Geometry check sheet. Reference: the model listing, model coordinates, mm. A direction names the side the tool comes from. Give positions to 0.01 mm unless a question says otherwise; leave off trailing zeros. Loops run counter-clockwise (first coordinate to the right, second up) from the corner with the lowest first, then second, coordinate; pieces in that order, holes last. Notation, with made-up numbers: (-26, 38.25) -> (22, 38.25) arc R11 ccw to (22, 52.25) -> close; hole circle Ø3 at (81, -34). An arc over 180 degrees is marked (long way). Write each question's results on one line, items separated by ' | '. Start each with the question number.
1) Sectioned sample at B-B on x = -2.5. Record the cut outline in (y, z).
2) Set-up check for faces 1 (the face through (3, 8, 6)), 2 (the face through (-3, 40.514, 6)), 3 (the face through (-3, 40.514, -6)), 4 (the face through (3, 40.514, 6)): record each of +Z, -Z, +X, -X, +Y, -Y from which the full face is reachable in a straight line by a thin tool's end or side.
3) Depth check by flat-ended pin: pin 1 (3 mm diameter, centred on y = 41.5, z = 1, fed in from +X); pin 2 (1 mm diameter, centred on x = -5.5, y = 10.5, fed in from +Z); pin 3 (3 mm diameter, centred on y = 24.5, z = 4.5, fed in from -X). Enter the tip coordinate at first touch or a pass-through.
4) Scan lines: line 1 (X direction, y = 38, z = -4.5); line 2 (X direction, y = 43, z = -3.5); line 3 (Z direction, x = 4.5, y = 7). Record each from-to range of solid material in increasing order. Write a range as from..to.
5) Sectioned sample at A-A on z = -2.5. Record the cut outline in (x, y), then the cut area to 3 significant figures.
6) Sectioned sample at C-C on y = 22. Record the cut outline in (x, z).
Autodesk Inventor part; units mm, degrees
ref_plane "Work Plane2" through (0, 24.257, 0) normal (0, 1, 0) x (1, 0, 0)
ref_plane "YZ Plane" through (0, 0, 0) normal (1, 0, 0) x (0, 1, 0)
ref_plane "XZ Plane" through (0, 0, 0) normal (0, 1, 0) x (-1, 0, 0)
sketch "Sketch1" plane through (0, 0, 0) normal (0, 1, 0) x (-1, 0, 0)
  line L0 (7.3323, 0) -> (3.6662, -6.35)
  line L1 (3.6662, -6.35) -> (-3.6662, -6.35)
  line L2 (-3.6662, -6.35) -> (-7.3323, 0)
  line L3 (-7.3323, 0) -> (-3.6662, 6.35)
  line L4 (-3.6662, 6.35) -> (3.6662, 6.35)
  line L5 (3.6662, 6.35) -> (7.3323, 0)
  line L6 (7.3323, 0) -> (0, 0)
  line L7 (0, 0) -> (0, -3.7196)
  dimension "d0" = 90
  dimension "d1" = 12.7
extrude "Extrusion1" add sketch "Sketch1" along normal blind 48.514
ref_plane "Work Plane2" through (0, 24.257, 0) normal (0, 1, 0) x (1, 0, 0)
sketch "Sketch3" plane through (0, 48.514, 0) normal (0, 1, 0) x (1, 0, 0)
  circle A0 centre (0, 0) radius 6.35
  line L0 (-3.6662, 6.35) -> (-7.3323, 0)
  line L1 (-3.6662, 6.35) -> (-7.3323, 0)
  line L2 (-7.3323, 0) -> (-3.6662, -6.35)
  line L3 (-3.6662, -6.35) -> (3.6662, -6.35)
  line L4 (3.6662, -6.35) -> (7.3323, 0)
  line L5 (7.3323, 0) -> (3.6662, 6.35)
  line L6 (3.6662, 6.35) -> (-3.6662, 6.35)
  dimension "d7" = 12.7
extrude "Extrusion3" cut sketch "Sketch3" against normal blind 8 contours A0 L5 L4 | A0 L6 L5 | L4 L3 A0 | A0 L0 L6 | L3 L2 A0 | A0 L2 L0
mirror "Mirror2" about plane through (0, 24.257, 0) normal (0, 1, 0) of "Extrusion3"
properties part number "Hex Shaft for E gear box"
Result:
1) outline: (0, -5.84) -> (8, -5.84) -> (8, -6.35) -> (40.51, -6.35) -> (40.51, -5.84) -> (48.51, -5.84) -> (48.51, 5.84) -> (40.51, 5.84) -> (40.51, 6.35) -> (8, 6.35) -> (8, 5.84) -> (0, 5.84) -> close
2) face 1: +Z, +X, -Y | face 2: +Z, -X, +Y | face 3: -Z, -X, +Y | face 4: +Z, +X, +Y
3) pin 1: x = 7.33 | pin 2: z = 4.04 | pin 3: x = -5.6
4) line 1: -4.73..4.73 | line 2: -5.3..5.3 | line 3: -4.48..4.48
5) outline: (-5.89, 8) -> (-5.84, 8) -> (-5.84, 0) -> (5.84, 0) -> (5.84, 8) -> (5.89, 8) -> (5.89, 40.51) -> (5.84, 40.51) -> (5.84, 48.51) -> (-5.84, 48.51) -> (-5.84, 40.51) -> (-5.89, 40.51) -> close | area: 570 mm^2
6) outline: (-7.33, 0) -> (-3.67, -6.35) -> (3.67, -6.35) -> (7.33, 0) -> (3.67, 6.35) -> (-3.67, 6.35) -> close
